from build123d import *

# Parameters (mm, degrees)
SKETCH1_W           = 127
SKETCH1_H           = 43.942
BOSS_EXTRUDE1_DEPTH = 10.16
SKETCH2_W           = 114.3
SKETCH2_H           = 33.782
SKETCH2_W_2         = 6.35
CUT_EXTRUDE1_DEPTH  = 8.89
CHAMFER1_SIZE       = 5.08
FILLET1_R           = 12.7
FILLET2_R           = 1.27


# Some blends are built 0.0001 mm under size
with BuildPart() as part:
    # Sketch1 → Boss-Extrude1 (new body)
    with BuildSketch(Plane(origin=(0, 0, 0), x_dir=(1, 0, 0), z_dir=(0, 1, 0))):
        Rectangle(SKETCH1_W, SKETCH1_H)
    extrude(amount=BOSS_EXTRUDE1_DEPTH)

    # Sketch2 → Cut-Extrude1 (cut)
    with BuildSketch(Plane(origin=(0, 10.16, 0), x_dir=(1, 0, 0), z_dir=(0, 1, 0))):
        Rectangle(SKETCH2_W, SKETCH2_H)
        with Locations((60.325, 0)):
            Rectangle(SKETCH2_W_2, SKETCH2_H)
        with Locations((-60.325, 0)):
            Rectangle(SKETCH2_W_2, SKETCH2_H)
    extrude(amount=-CUT_EXTRUDE1_DEPTH, mode=Mode.SUBTRACT)

    # Chamfer1
    chamfer1_edges = [part.edges().sort_by_distance(p)[0] for p in [
        (0, 10.16, 16.891),
        (0, 10.16, -16.891),
    ]]
    chamfer(chamfer1_edges, length=CHAMFER1_SIZE - 0.0001)  # a hair under: the kernel refuses the full size

    # Fillet1
    # the kernel refuses this fillet: 12.7 mm, written as the material it takes off along each edge
    with BuildSketch(Plane(origin=(76.317910379, 5.0801, 16.891), x_dir=(0, -1, 0), z_dir=(-1, 0, 0))) as fillet1_piece_1:
        with BuildLine():
            CenterArc((5.354803581, 12.605708661), FILLET1_R, 225, 38.013804416)
            Line((-3.62545254, 3.62545254), (-3.805057662, 3.445847418))
            Line((-3.805057662, 3.445847418), (-0.179605122, -0.179605122))
            Line((-0.179605122, -0.179605122), (0, -0.254))
            ThreePointArc((0, -0.254), (1.90505, -0.254), (3.779205928, -0.252114173))
            Line((3.779205928, -0.252114173), (3.8101, 0))
        make_face()
    extrude(amount=152.635820759, mode=Mode.SUBTRACT)
    with BuildSketch(Plane(origin=(76.317910379, 5.0801, -16.891), x_dir=(0, 0.7071067811865474, -0.7071067811865477), z_dir=(-1, 0, 0))) as fillet1_piece_2:
        with BuildLine():
            CenterArc((5.127164152, 12.7), FILLET1_R, 231.986195584, 38.013804416)
            Line((-2.694147547, 2.694147547), (-2.850573781, 2.494030498))
            ThreePointArc((-2.850573781, 2.494030498), (-1.526678896, 1.167468651), (-0.179605122, -0.179605122))
            Line((-0.179605122, -0.179605122), (0, -0.254))
            Line((0, -0.254), (5.127164152, -0.254))
            Line((5.127164152, -0.254), (5.127164152, 0))
        make_face()
    extrude(amount=152.635820759, mode=Mode.SUBTRACT)

    # Fillet2
    fillet2_edges = [part.edges().sort_by_distance(p)[0] for p in [
        (0, 1.27, 16.891),
        (0, 1.27, -16.891),
    ]]
    fillet(fillet2_edges, radius=FILLET2_R)


solid = part.part
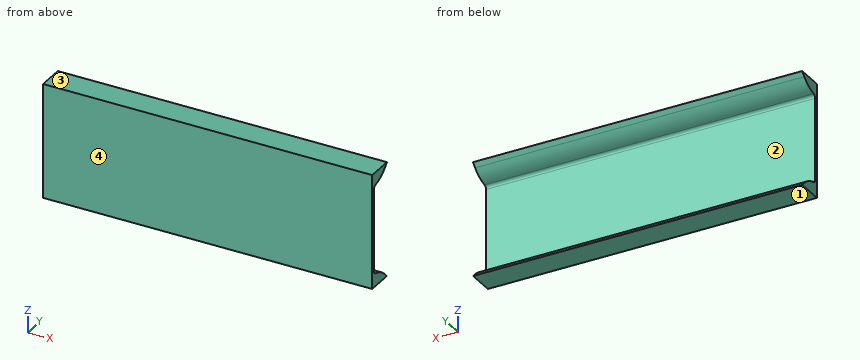
Model file for the job. Use its own axes, mm. Face numbers are marked on the shaded views. Give positions to 0.01 mm unless a question says otherwise; leave off trailing zeros. Order: outer loops, then holes, each group sorted by start corner. A loop starts at its lowest first (then second) coordinate and runs counter-clockwise, first axis right, second up. Notation, with made-up numbers: (32, 72) - (40, 72) arc R23 ccw to (40, 100) - close; hole circle Ø6 at (21.25, 48.5). An arc over 180 degrees is marked (long way). One line per item, written item: value.
Item 1: Two-plate mould, pull along Z, no slides. Class the marked faces 1, 2, 3 and 4: released by +Z, released by -Z, zero draft, split by the parting line, or undercut.
Response values:
face 1: released by -Z
face 2: undercut
face 3: released by +Z
face 4: zero draft
Item 2: Slice it at C-C (z = -14). List the corners of the cut face in (x, y), then the cut area to 3 significant figures.
Response values:
outline: (-63.5, 0) - (63.5, 0) - (63.5, 1.27) - (-63.5, 1.27) - close
area: 161 mm2
Item 3: Slice it at A-A (y = 4.5). List the corners of the cut face in (x, z).
Response values:
outline: (-63.5, -21.97) - (63.5, -21.97) - (63.5, -17.73) - (-63.5, -17.73) - close; (-63.5, 17.73) - (63.5, 17.73) - (63.5, 21.97) - (-63.5, 21.97) - close
Item 4: Wall check: line 1 (Y direction, x = -24.5, z = -8); line 2 (Z direction, x = -50.5, y = 9); line 3 (Z direction, x = -55, y = 4.75). Give the ranges that are in metal, low to high.
Response values:
line 1: 0 to 1.27
line 2: -21.97 to -20.81, 20.81 to 21.97
line 3: -21.97 to -17.83, 17.83 to 21.97
Item 5: Pin check, flat tips, straight feed: pin 1 Ø6 at (y, z) = (4.5, -3.5) entering from +X; pin 2 Ø5 at (x, z) = (10, 1.5) entering from -Y; pin 3 Ø16 at (x, z) = (-29.5, 3) entering from +Y. Stop position of each tip, or through.
Response values:
pin 1: through
pin 2: y = 0
pin 3: y = 1.27
